Here's how the part is built. I have some questions about the finished solid (model axes, mm). Face numbers are marked on the shaded views. A direction names the side the tool comes from. Round coordinates to 2 decimals unless told otherwise and drop trailing zeros. Order: outer loops, then holes, each group sorted by start corner. A loop starts at its lowest first (then second) coordinate and runs counter-clockwise, first axis right, second up. Notation, with made-up numbers: (47.25, 37.25) - (72.25, 37.25) arc R24 ccw to (72.25, 68.25) - close; hole circle Ø1 at (58.25, 69.25). An arc over 180 degrees is marked (long way). Answer as a JSON object with one key per item and string values.
```python
from build123d import *

# Parameters (mm, degrees)
SKETCH1_W           = 30
SKETCH1_H           = 36
BOSS_EXTRUDE1_DEPTH = 30
SKETCH3_R           = 12.375
CUT_EXTRUDE1_DEPTH  = 40
SKETCH5_R           = 1.875
CUT_EXTRUDE2_DEPTH  = 40
CUT_EXTRUDE3_START  = 15
SKETCH7_W           = 36
SKETCH7_H           = 15
CUT_EXTRUDE3_DEPTH  = 31
SKETCH8_W           = 5.625
SKETCH8_H           = 15
BOSS_EXTRUDE2_DEPTH = 7
SKETCH10_W          = 24.75
SKETCH10_H          = 15
BOSS_EXTRUDE3_DEPTH = 3
SKETCH11_W          = 36
SKETCH11_H          = 5.8
SKETCH11_H_2        = 2
BOSS_EXTRUDE4_DEPTH = 8
SKETCH12_W          = 8
SKETCH12_H          = 36
CUT_EXTRUDE4_DEPTH  = 3
SKETCH13_R          = 1
CUT_EXTRUDE5_DEPTH  = 3


with BuildPart() as part:
    # Sketch1 → Boss-Extrude1 (new body)
    with BuildSketch(Plane(origin=(0, 0, 0), x_dir=(1, 0, 0), z_dir=(0, 1, 0))):
        Rectangle(SKETCH1_W, SKETCH1_H)
    extrude(amount=BOSS_EXTRUDE1_DEPTH)

    # Sketch3 → Cut-Extrude1 (cut)
    with BuildSketch(Plane(origin=(15, 0, 0), x_dir=(0, 0, -1), z_dir=(1, 0, 0))):
        with Locations((0, 15)):
            Circle(SKETCH3_R)
    extrude(amount=-CUT_EXTRUDE1_DEPTH, mode=Mode.SUBTRACT)

    # Sketch5 → Cut-Extrude2 (cut)
    with BuildSketch(Plane(origin=(0, 30, 0), x_dir=(1, 0, 0), z_dir=(0, 1, 0))):
        with Locations((-12.25, 15.25)):
            Circle(SKETCH5_R)
        with Locations((-12.25, -15.25)):
            Circle(SKETCH5_R)
        with Locations((12.25, -15.25)):
            Circle(SKETCH5_R)
        with Locations((12.25, 15.25)):
            Circle(SKETCH5_R)
    extrude(amount=-CUT_EXTRUDE2_DEPTH, mode=Mode.SUBTRACT)

    # Sketch7 → Cut-Extrude3 (cut, through all)
    with BuildSketch(Plane(origin=(0, 0, 0), x_dir=(0, 0, -1), z_dir=(1, 0, 0)).offset(CUT_EXTRUDE3_START)):
        with Locations((0, 7.5)):
            Rectangle(SKETCH7_W, SKETCH7_H)
    extrude(amount=-CUT_EXTRUDE3_DEPTH, mode=Mode.SUBTRACT)

    # Sketch8 → Boss-Extrude2 (add)
    with BuildSketch(Plane(origin=(15, 0, 0), x_dir=(0, 0, -1), z_dir=(1, 0, 0))):
        with Locations((-15.1875, 22.5)):
            Rectangle(SKETCH8_W, SKETCH8_H)
        with Locations((15.1875, 22.5)):
            Rectangle(SKETCH8_W, SKETCH8_H)
    extrude(amount=BOSS_EXTRUDE2_DEPTH)

    # Sketch10 → Boss-Extrude3 (add)
    with BuildSketch(Plane(origin=(22, 0, 0), x_dir=(0, 0, -1), z_dir=(1, 0, 0))):
        with Locations((0, 22.5)):
            Rectangle(SKETCH10_W, SKETCH10_H)
    extrude(amount=-BOSS_EXTRUDE3_DEPTH)

    # Sketch11 → Boss-Extrude4 (add)
    with BuildSketch(Plane(origin=(22, 0, 0), x_dir=(0, 0, -1), z_dir=(1, 0, 0))):
        with Locations((0, 27.1)):
            Rectangle(SKETCH11_W, SKETCH11_H)
        with Locations((0, 16)):
            Rectangle(SKETCH11_W, SKETCH11_H_2)
    extrude(amount=BOSS_EXTRUDE4_DEPTH)

    # Sketch12 → Cut-Extrude4 (cut)
    with BuildSketch(Plane(origin=(0, 30, 0), x_dir=(1, 0, 0), z_dir=(0, 1, 0))):
        with Locations((26, 0)):
            Rectangle(SKETCH12_W, SKETCH12_H)
    extrude(amount=-CUT_EXTRUDE4_DEPTH, mode=Mode.SUBTRACT)

    # Sketch13 → Cut-Extrude5 (cut)
    with BuildSketch(Plane(origin=(0, 27, 0), x_dir=(1, 0, 0), z_dir=(0, 1, 0))):
        with Locations((25.64, 4)):
            Circle(SKETCH13_R)
        with Locations((25.64, -4)):
            Circle(SKETCH13_R)
    extrude(amount=-CUT_EXTRUDE5_DEPTH, mode=Mode.SUBTRACT)


solid = part.part
```
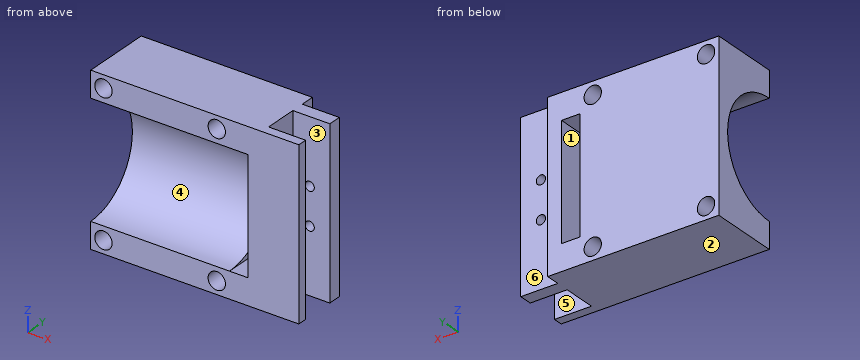
1. Imagine slicing it at C-C (x = -3.5). List the corners of the cut face in (y, z) for me (3 decimals), plus the area to 3 significant figures.
Responses:
{"outline": "(15, -18) - (30, -18) - (30, 18) - (15, 18) - (15, 12.375) arc R12.375 cw to (15, -12.375) - close", "area": "299 mm2"}
2. Imagine slicing it at A-A (z = 15.25). List the corners of the cut face in (x, y) for me (3 decimals), plus the area to 3 significant figures.
Responses:
{"outline": "(-15, 15) - (-14.125, 15) - (-14.125, 30) - (-15, 30) - close; (-10.375, 15) - (10.375, 15) - (10.375, 30) - (-10.375, 30) - close; (14.125, 15) - (30, 15) - (30, 17) - (22, 17) - (22, 24.2) - (30, 24.2) - (30, 27) - (22, 27) - (22, 30) - (14.125, 30) - close", "area": "481 mm2"}
3. If I drill on L1, parallel to X at y = 18.75, z = 15.25 (3 decimals); L2, parallel to X at y = 26.25, z = -15.25 (3 decimals); L3, parallel to Z at x = 25.64, y = 26.4, over which ranges is the centre line in solid material (lowest first)? Write a range as [from, to].
Responses:
{"L1": "[-15, -14.125], [-10.375, 10.375], [14.125, 22]", "L2": "[-15, -14.125], [-10.375, 10.375], [14.125, 30]", "L3": "[-18, -5], [-3, 3], [5, 18]"}
4. Thinking about a two-plate mould opening in Z: for the marked faces 1, 2 and 3, which applies, pulls with the +Z half, pulls with the -Z half, needs draft (parallel to the pull), parting line crosses it, or undercut?
Responses:
{"face 1": "undercut", "face 2": "pulls with the -Z half", "face 3": "needs draft"}
5. For P1, Ø4, axis at x = 26.5, z = 6.5, coming from the +Y side; P2, Ø3.5, axis at y = 19.5, z = -3, coming from the +X side; P3, Ø3, axis at y = 17.5, z = 8, coming from the -X side; P4, Ø5, axis at x = 24, y = 21.5, coming from the -Z side, each with a flat end and sliding along its axis, tell me the tip position at first contact or that it passes through.
Responses:
{"P1": "y = 27", "P2": "x = 22", "P3": "x = 19", "P4": "z = -18"}
6. Imagine slicing it at B-B (y = 19.5). List the corners of the cut face in (x, z) for me (3 decimals).
Responses:
{"outline": "(-15, -18) - (22, -18) - (22, 18) - (-15, 18) - (-15, 11.528) - (15, 11.528) - (15, 12.375) - (19, 12.375) - (19, -12.375) - (15, -12.375) - (15, -11.528) - (-15, -11.528) - close; hole circle Ø3.75 at (-12.25, -15.25); hole circle Ø3.75 at (-12.25, 15.25); hole circle Ø3.75 at (12.25, -15.25); hole circle Ø3.75 at (12.25, 15.25)"}
7. Imagine slicing it at D-D (y = 26). List the corners of the cut face in (x, z) for me (3 decimals), plus the area to 3 significant figures.
Responses:
{"outline": "(-15, -18) - (30, -18) - (30, 18) - (-15, 18) - (-15, 5.669) - (15, 5.669) - (15, 12.375) - (19, 12.375) - (19, -12.375) - (15, -12.375) - (15, -5.669) - (-15, -5.669) - close; hole circle Ø3.75 at (-12.25, -15.25); hole circle Ø3.75 at (-12.25, 15.25); hole circle Ø3.75 at (12.25, -15.25); hole circle Ø3.75 at (12.25, 15.25); hole circle Ø2 at (25.64, -4); hole circle Ø2 at (25.64, 4)", "area": "1,130 mm2"}
8. For the marked faces 4, 5 and 6, which set-ups out of +Z, -Z, +X, -X, +Y, -Y let a thin tool reach every point of the face, with its end or its side?
Responses:
{"face 4": "-X, -Y", "face 5": "+Z, -Z, +X", "face 6": "+Z, -Z, +X, +Y"}
